Design review of the part built by this model. Coordinates are the model's own, in mm. Coordinates: 2 decimals unless noted, no trailing zeros. Write each loop counter-clockwise with the first axis right and the second up, starting at its lowest first coordinate (ties: lowest second). Pieces come first, ordered by that corner, then holes. Notation, with made-up numbers: (16, 56.5) - (31, 56.5) arc R17 cw to (31, 62.5) - close; hole circle Ø8 at (-39, 24). An arc over 180 degrees is marked (long way). Answer as a JSON object with one key per item and string values.
```python
from build123d import *

# Parameters (mm, degrees)
MAIN_DEPTH               = 5.13
SKETCH2_R                = 1.5
SKETCH2_W                = 5.13
SKETCH2_H                = 58.88
CUT_EXTRUDE1_DEPTH       = 5.13
TOOTH_SLOT_REACH         = 7.13
SKETCH3_W                = 58.88
SKETCH3_H                = 5.13
LPATTERN1_COUNT          = 2
LPATTERN1_PITCH          = 118.88
LPATTERN1_COUNT_DIR2     = 2
LPATTERN1_PITCH_DIR2     = 114.36
M3_CLEARANCE_HOLE4_D     = 3.2
M3_CLEARANCE_HOLE4_DEPTH = 5.1
M3_CLEARANCE_HOLE4_TIP   = 0.96137699


with BuildPart() as part:
    # Sketch1 → Main (new body)
    with BuildSketch(Plane(origin=(0, 0, 0), x_dir=(1, 0, 0), z_dir=(0, 1, 0))):
        with BuildLine():
            Line((-55.207201859, 101.249932113), (117.542798141, 101.249932113))
            ThreePointArc((117.542798141, 101.249932113), (126.523054262, 97.530188234), (130.242798141, 88.549932113))
            Line((130.242798141, 88.549932113), (130.242798141, -19.530067887))
            ThreePointArc((130.242798141, -19.530067887), (126.523054262, -28.510324008), (117.542798141, -32.230067887))
            Line((117.542798141, -32.230067887), (-55.207201859, -32.230067887))
            ThreePointArc((-55.207201859, -32.230067887), (-64.18745798, -28.510324008), (-67.907201859, -19.530067887))
            Line((-67.907201859, -19.530067887), (-67.907201859, 88.549932113))
            ThreePointArc((-67.907201859, 88.549932113), (-64.18745798, 97.530188234), (-55.207201859, 101.249932113))
        make_face()
    extrude(amount=MAIN_DEPTH)

    # Sketch2 → Cut-Extrude1 (cut)
    with BuildSketch(Plane(origin=(0, 5.13, 0), x_dir=(1, 0, 0), z_dir=(0, 1, 0))):
        with Locations((-58.347201859, -14.930067887)):
            Circle(SKETCH2_R)
        with Locations((-58.347201859, 83.949932113)):
            Circle(SKETCH2_R)
        with Locations((120.682798141, 83.949932113)):
            Circle(SKETCH2_R)
        with Locations((120.682798141, -14.930067887)):
            Circle(SKETCH2_R)
        with Locations((-58.342201859, 34.509932113)):
            Rectangle(SKETCH2_W, SKETCH2_H)
        with Locations((120.677798141, 34.509932113)):
            Rectangle(SKETCH2_W, SKETCH2_H)
    extrude(amount=-CUT_EXTRUDE1_DEPTH, mode=Mode.SUBTRACT)

    # Sketch3 → tooth slot (cut, up to next)
    with BuildSketch(Plane(origin=(0, 5.13, 0), x_dir=(1, 0, 0), z_dir=(0, 1, 0)), mode=Mode.PRIVATE) as tooth_slot_sk1:
        with Locations((31.167798141, -22.665067887)):
            Rectangle(SKETCH3_W, SKETCH3_H)
    tooth_slot_tool1 = extrude(tooth_slot_sk1.sketch, amount=-TOOTH_SLOT_REACH, mode=Mode.PRIVATE) & part.part
    add(tooth_slot_tool1.solids().sort_by_distance((31.167798, 5.13, 22.665068))[0], mode=Mode.SUBTRACT)

    # Sketch4 → M3 Clearance Hole1 (revolve, cut)
    with BuildSketch(Plane(origin=(-28.272201859, 5.13, 22.401258672), x_dir=(0, 0, 1), z_dir=(1, 0, 0))):
        Polygon((0, 0), (0, 6.06137699), (1.6, 5.1), (1.6, 0), align=None)
    m3_clearance_hole1 = revolve(axis=Axis((-28.272201859, 11.48, 22.401258672), (0, -1, 0)), mode=Mode.SUBTRACT)

    # LPattern1: M3 Clearance Hole1 2 × 2
    with Locations(*[(i * LPATTERN1_PITCH, 0, -j * LPATTERN1_PITCH_DIR2) for i in range(LPATTERN1_COUNT) for j in range(LPATTERN1_COUNT_DIR2) if (i, j) != (0, 0)]):
        add(m3_clearance_hole1, mode=Mode.SUBTRACT)

    # M3 Clearance Hole4
    with Locations(Plane(origin=(0, 5.13, 0), x_dir=(-1, 0, 0), z_dir=(0, 1, 0))):
        with Locations((-100.998782657, -48.960031461), (-106.146516037, 3.363968539), (-57.818782657, 2.039968539), (-26.068782657, -27.170031461)):
            Hole(M3_CLEARANCE_HOLE4_D / 2, depth=M3_CLEARANCE_HOLE4_DEPTH)
            with Locations((0, 0, -(M3_CLEARANCE_HOLE4_DEPTH + M3_CLEARANCE_HOLE4_TIP / 2))):  # 118° drill point
                Cone(0, M3_CLEARANCE_HOLE4_D / 2, M3_CLEARANCE_HOLE4_TIP, mode=Mode.SUBTRACT)


solid = part.part
```
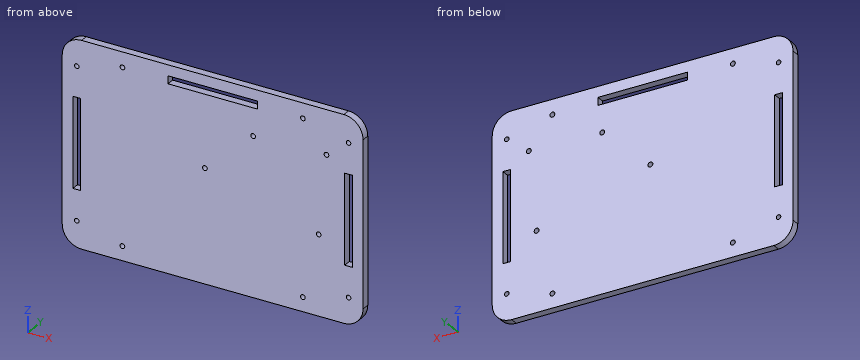
(1) Take a section at C-C, the plane y = 3.1. Give the number of separate pieces and of enclosed holes in the cut face, and give its area (3 significant figures).
Solved:
{"separate pieces": "1", "enclosed holes": "15", "area": "25,300 mm^2"}
(2) For pin 1 (4 mm diameter, centred on x = 57.82, z = 2.04, fed in from -Y); pin 2 (1.5 mm diameter, centred on x = -57, y = 1.5, fed in from +Z); pin 3 (2.5 mm diameter, centred on x = 120.68, z = 14.93, fed in from -Y), all flat-tipped, find the tip position at first contact; note any pin that passes through.
Solved:
{"pin 1": "stops at y = 0", "pin 2": "stops at z = 32.19", "pin 3": "passes through"}
(3) Take a section at B-B, the plane z = -58. Write out the cut boundary in (x, y), and give its area (3 significant figures).
Solved:
{"outline": "(-67.91, 0) - (-60.91, 0) - (-60.91, 5.13) - (-67.91, 5.13) - close; (-55.78, 0) - (118.11, 0) - (118.11, 5.13) - (-55.78, 5.13) - close; (123.24, 0) - (130.24, 0) - (130.24, 5.13) - (123.24, 5.13) - close", "area": "964 mm^2"}
(4) To check wall thickness, follow line 1 (X direction, y = 1.4, z = -13); line 2 (Z direction, x = 37, y = 2); line 3 (Z direction, x = 118.5, y = 4.25). State the ranges of each line that lie inside material, in increasing order. Write a range as from..to.
Solved:
{"line 1": "x = -67.91..-60.91, -55.78..118.11, 123.24..130.24", "line 2": "z = -101.25..20.1, 25.23..32.23", "line 3": "z = -101.21..-63.95, -5.07..32.19"}
(5) Take a section at A-A, the plane x = 49. Write out the cut boundary in (y, z), and give its area (3 significant figures).
Solved:
{"outline": "(0, -101.25) - (5.13, -101.25) - (5.13, 20.1) - (0, 20.1) - close; (0, 25.23) - (5.13, 25.23) - (5.13, 32.23) - (0, 32.23) - close", "area": "658 mm^2"}
